```python
from build123d import *

# Parameters (mm, degrees)
SKETCH3_R          = 1.5
BASE_DEPTH         = 7
WALLS_START        = 7
SKETCH3_3_R        = 1.5
WALLS_DEPTH        = 23
STANDOFFS_START    = 7
SKETCH3_4_R        = 2.5
SKETCH3_4_R_2      = 1.5
STANDOFFS_DEPTH    = 3
INTERNAL_FILLET_R  = 3
EXTERNAL_FILLET_R  = 3
SKETCH5_R          = 7.9
CUT_EXTRUDE1_DEPTH = 10


# Some blends are built 0.0001 mm under size
with BuildPart() as part:
    # Sketch3 → base (new body)
    with BuildSketch(Plane.XY):
        with BuildLine():
            ThreePointArc((-4.5, 74.5), (-7, 72), (-4.5, 69.5))
            Line((-4.5, 69.5), (-2, 69.5))
            Line((-2, 69.5), (-2, 0))
            ThreePointArc((-2, 0), (-1.414213562, -1.414213562), (0, -2))
            Line((0, -2), (40, -2))
            ThreePointArc((40, -2), (41.414213562, -1.414213562), (42, 0))
            Line((42, 0), (42, 5.5))
            Line((42, 5.5), (44.5, 5.5))
            ThreePointArc((44.5, 5.5), (47, 8), (44.5, 10.5))
            Line((44.5, 10.5), (42, 10.5))
            Line((42, 10.5), (42, 80))
            ThreePointArc((42, 80), (41.414213562, 81.414213562), (40, 82))
            Line((40, 82), (0, 82))
            ThreePointArc((0, 82), (-1.414213562, 81.414213562), (-2, 80))
            Line((-2, 80), (-2, 74.5))
            Line((-2, 74.5), (-4.5, 74.5))
        make_face()
        with Locations((44.5, 8)):
            Circle(SKETCH3_R, mode=Mode.SUBTRACT)
        with Locations((-4.5, 72)):
            Circle(SKETCH3_R, mode=Mode.SUBTRACT)
    extrude(amount=BASE_DEPTH)

    # Sketch3<3> → walls (add)
    with BuildSketch(Plane.XY.offset(WALLS_START)):
        with BuildLine():
            Line((-2, 74.5), (-2, 69.5))
            Line((-2, 69.5), (-2, 0))
            ThreePointArc((-2, 0), (-1.414213562, -1.414213562), (0, -2))
            Line((0, -2), (40, -2))
            ThreePointArc((40, -2), (41.414213562, -1.414213562), (42, 0))
            Line((42, 0), (42, 5.5))
            Line((42, 5.5), (42, 10.5))
            Line((42, 10.5), (42, 80))
            ThreePointArc((42, 80), (41.414213562, 81.414213562), (40, 82))
            Line((40, 82), (0, 82))
            ThreePointArc((0, 82), (-1.414213562, 81.414213562), (-2, 80))
            Line((-2, 80), (-2, 74.5))
        make_face()
        with BuildLine():
            ThreePointArc((0.00181331, 1.914853357), (1.366810234, 1.724189535), (2, 0.5))
            ThreePointArc((2, 0.5), (1.978560116, 0.247294673), (1.914853357, 0.00181331))
            ThreePointArc((1.914853357, 0.00181331), (-0.560660172, -0.560660172), (0.00181331, 1.914853357))
        make_face(mode=Mode.SUBTRACT)
        with Locations((39.5, 0.5)):
            Circle(SKETCH3_3_R, mode=Mode.SUBTRACT)
        with Locations((0.5, 79.5)):
            Circle(SKETCH3_3_R, mode=Mode.SUBTRACT)
        with BuildLine():
            ThreePointArc((0, 77.050510257), (2.267766953, 77.732233047), (2.949489743, 80))
            Line((2.949489743, 80), (37.050510257, 80))
            ThreePointArc((37.050510257, 80), (37.732233047, 77.732233047), (40, 77.050510257))
            Line((40, 77.050510257), (40, 2.949489743))
            ThreePointArc((40, 2.949489743), (37.732233047, 2.267766953), (37.050510257, 0))
            Line((37.050510257, 0), (2.949489743, 0))
            ThreePointArc((2.949489743, 0), (2.267766953, 2.267766953), (0, 2.949489743))
            Line((0, 2.949489743), (0, 77.050510257))
        make_face(mode=Mode.SUBTRACT)
        with Locations((39.5, 79.5)):
            Circle(SKETCH3_3_R, mode=Mode.SUBTRACT)
    extrude(amount=WALLS_DEPTH)

    # Sketch3<4> → standoffs (add)
    # profile 1 of 2: a face of its own
    with BuildSketch(Plane.XY.offset(STANDOFFS_START)):
        with Locations((20, 49.5)):
            Circle(SKETCH3_4_R)
        with Locations((20, 49.5)):
            Circle(SKETCH3_4_R_2, mode=Mode.SUBTRACT)
    # profile 2 of 2: a face of its own
    with BuildSketch(Plane.XY.offset(STANDOFFS_START)):
        with Locations((20, 9)):
            Circle(SKETCH3_4_R)
        with Locations((20, 9)):
            Circle(SKETCH3_4_R_2, mode=Mode.SUBTRACT)
    extrude(amount=STANDOFFS_DEPTH)

    # Internal Fillet
    internal_fillet_edges = [part.edges().sort_by_distance(p)[0] for p in [
        (17.5, 49.5, 7),
        (17.5, 9, 7),
        (40, 40, 7),
        (20, 80, 7),
        (0, 40, 7),
        (0, 2.949489743, 18.5),
        (2.267766953, 2.267766953, 7),
        (2.949489743, 0, 18.5),
        (20, 0, 7),
        (37.050510257, 0, 18.5),
        (37.732233047, 2.267766953, 7),
        (40, 2.949489743, 18.5),
        (40, 77.050510257, 18.5),
        (37.732233047, 77.732233047, 7),
        (37.050510257, 80, 18.5),
        (2.949489743, 80, 18.5),
        (2.267766953, 77.732233047, 7),
        (0, 77.050510257, 18.5),
    ]]
    fillet(internal_fillet_edges, radius=INTERNAL_FILLET_R - 0.0001)  # a hair under: the kernel refuses the full size

    # External Fillet
    # the kernel refuses this fillet: 3 mm, written as the material it adds along each edge
    with BuildSketch(Plane(origin=(42, 5.5, 0), x_dir=(0, -1, 0), z_dir=(0, 0, 1)), Plane(origin=(-2, 74.5, 0), x_dir=(0, 1, 0), z_dir=(0, 0, 1))) as external_fillet_piece_1:
        with BuildLine():
            CenterArc((2.977225575, 3), EXTERNAL_FILLET_R, 185.21590857, 84.78409143)
            Line((-0.010352011, 2.727272727), (-0.30910977, 2.7))
            ThreePointArc((-0.30910977, 2.7), (-0.3, 2.5), (-0.3, 0))
            Line((-0.3, 0), (0, -0.3))
            Line((0, -0.3), (2.977225575, -0.3))
            Line((2.977225575, -0.3), (2.977225575, 0))
        make_face()
    extrude(amount=7)
    with BuildSketch(Plane(origin=(42, 10.5, 0), x_dir=(0, 1, 0), z_dir=(0, 0, 1)), Plane(origin=(-2, 69.5, 0), x_dir=(0, -1, 0), z_dir=(0, 0, 1))) as external_fillet_piece_2:
        with BuildLine():
            CenterArc((2.977225575, -3), EXTERNAL_FILLET_R, 90, 84.78409143)
            Line((-0.010352011, -2.727272727), (-0.30910977, -2.7))
            ThreePointArc((-0.30910977, -2.7), (-0.3, -2.5), (-0.3, 0))
            Line((-0.3, 0), (0, 0.3))
            Line((0, 0.3), (2.977225575, 0.3))
            Line((2.977225575, 0.3), (2.977225575, 0))
        make_face()
    extrude(amount=7)

    # Sketch5 → Cut-Extrude1 (cut)
    with BuildSketch(Plane.ZY.offset(-40)):
        with Locations(Location((18.9, 65.168153045, 0), (0, 0, 270))):
            Circle(SKETCH5_R)
    extrude(amount=-CUT_EXTRUDE1_DEPTH, mode=Mode.SUBTRACT)


solid = part.part
```
CAD build for the part. Positions are in the model's coordinates, mm. A direction names the side the tool comes from. Coordinates: 2 decimals unless noted, no trailing zeros. Write each loop counter-clockwise with the first axis right and the second up, starting at its lowest first coordinate (ties: lowest second). Pieces come first, ordered by that corner, then holes.
(1) Cut at C-C, the plane y = 72. List the corners of the cut face in (x, z), and give its area (3 significant figures).
(2) Cut at D-D, the plane z = 12. Count the separate pieces of the cut face and the enclosed holes in it, and give its area (3 significant figures).
(3) Cut at A-A, the plane x = 27.5. List the corners of the cut face in (y, z), and give its area (3 significant figures).
(4) Flat gauge pins, fed straight in: pin 1 (1.5 mm diameter, centred on x = 3.5, y = 20, fed in from +Z); pin 2 (4 mm diameter, centred on x = 19.5, y = 50.5, fed in from +Z); pin 3 (1 mm diameter, centred on y = 16, z = 15.5, fed in from -X). Where does each tip first touch, or does it go through?
(5) Two-plate mould, pull along Y, no slides. Class faces 3 (the face through (20, 50, 7)), 4 (the face through (40.99, 57.63, 21.27)), 5 (the face through (43, 7, 7)), 6 (the face through (-1.4, 81.43, 14.79)): +Y half, -Y half, draft (parallel to the pull), parting line (faces both ways), or undercut.
(6) 3-axis set-ups, long thin cutter, end or side, ignore diameter. For faces 1 (the face through (43, 8, 3)), 2 (the face through (1.306, 80.765, 18.339)): which of +Z, -Z, +X, -X, +Y, -Y reach the whole face in a straight line?
(7) Drill centre lines: probe 1 along X at (y, z) = (40.5, 12.5); probe 2 along Y at (x, z) = (13, 22); probe 3 along Y at (x, z) = (39.5, 21.25). Where is each one in solid material? Low to high.
Geometry says:
1. outline: (-7, 0) - (-6, 0) - (-6, 7) - (-7, 7) - close; (-3, 0) - (42, 0) - (42, 14.93) - (40, 14.93) - (40, 10) arc R3 cw to (37, 7) - (3, 7) arc R3 cw to (0, 10) - (0, 30) - (-2, 30) - (-2, 7) - (-3, 7) - close; (40, 22.87) - (42, 22.87) - (42, 30) - (40, 30) - close
1. area: 402 mm2
2. separate pieces: 1
2. enclosed holes: 4
2. area: 487 mm2
3. outline: (-2, 0) - (82, 0) - (82, 30) - (80, 30) - (80, 10) arc R3 cw to (77, 7) - (3, 7) arc R3 cw to (0, 10) - (0, 30) - (-2, 30) - close
3. area: 684 mm2
4. pin 1: stops at z = 7.01
4. pin 2: stops at z = 10
4. pin 3: stops at x = -2
5. face 3: undercut
5. face 4: undercut
5. face 5: draft
5. face 6: +Y half
6. face 1: +Z, -Z
6. face 2: +Z
7. probe 1: x = -2 to 0, 40 to 42
7. probe 2: y = -2 to 0, 80 to 82
7. probe 3: y = -2 to -1, 2 to 3.74, 76.26 to 78, 81 to 82
